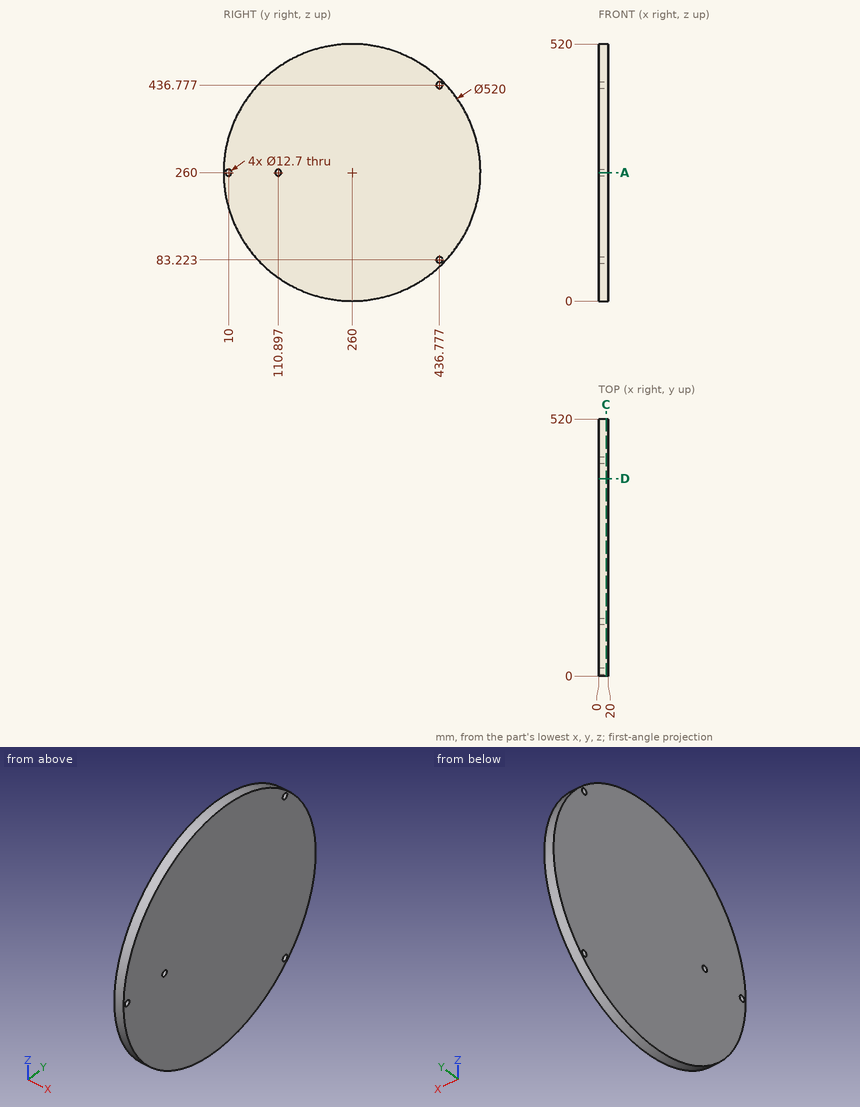
Could you check a few things on this drawing? It's one solid part, dimensions in mm from its lowest x, y, z. Coordinates: 2 decimals unless noted, no trailing zeros. Loops run counter-clockwise (first coordinate to the right, second up) from the corner with the lowest first, then second, coordinate; pieces in that order, holes last. Notation, with made-up numbers: (16.25, 78) - (41.25, 78) arc R17 cw to (41.25, 101) - close; hole circle Ø10 at (-5, -27). An arc over 180 degrees is marked (long way). Answer as a JSON object with one key per item and string values. Group by question number.
Item 1: If we section it at A-A (z = 260): List the corners of the cut face in (x, y) for me, plus the area to 3 significant figures.
Item 2: For pin 1 (8 mm diameter, centred on x = 15.5, z = 113, fed in from +Y); pin 2 (3 mm diameter, centred on x = 10, y = 439.5, fed in from +Z) (1 decimal); pin 3 (2 mm diameter, centred on x = 9, y = 62, fed in from +Z), each with a flat end and sliding along its axis, tell me the tip position at first contact or that it passes through.
Item 3: If we section it at D-D (y = 399.5): List the corners of the cut face in (x, z) for me.
Item 4: If I drill on L1, parallel to Y at x = 16, z = 260; L2, parallel to Z at x = 1.75, y = 223 (1 decimal); L3, parallel to Z at x = 16.25, y = 173, over which ranges is the centre line in solid material (lowest first)? Write a range as from..to.
Item 5: If we section it at C-C (x = 15.25): List the corners of the cut face in (y, z) for me.
Returned:
{
 "1": {"outline": "(0, 0) - (20, 0) - (20, 3.65) - (0, 3.65) - close; (0, 16.35) - (20, 16.35) - (20, 104.55) - (0, 104.55) - close; (0, 117.25) - (20, 117.25) - (20, 520) - (0, 520) - close", "area": "9,890 mm²"},
 "2": {"pin 1": "stops at y = 477.14", "pin 2": "stops at z = 449.5", "pin 3": "stops at z = 429.68"},
 "3": {"outline": "(0, 40.59) - (20, 40.59) - (20, 479.41) - (0, 479.41) - close"},
 "4": {"L1": "y = 0..3.65, 16.35..104.55, 117.25..520", "L2": "z = 2.6..517.4", "L3": "z = 14.99..505.01"},
 "5": {"outline": "circle Ø520 at (260, 260); hole circle Ø12.7 at (10, 260); hole circle Ø12.7 at (110.9, 260); hole circle Ø12.7 at (436.78, 83.22); hole circle Ø12.7 at (436.78, 436.78)"}
}
